Could you check a few things on this model? Use its own coordinates, in mm. Round coordinates to 2 decimals unless told otherwise and drop trailing zeros. Loops run counter-clockwise (first coordinate to the right, second up) from the corner with the lowest first, then second, coordinate; pieces in that order, holes last. Notation, with made-up numbers: (27.5, -7) -> (68.5, -7) arc R29 ccw to (68.5, 18) -> close; hole circle Ø8 at (-23.75, 33.5). An arc over 180 degrees is marked (long way). One line per item, written item: value.
```python
from build123d import *

# Parameters (mm, degrees)
SKETCH2_W           = 90
SKETCH2_H           = 92.5
SKETCH2_R           = 2
SKETCH2_W_2         = 10
SKETCH2_H_2         = 3
SKETCH2_W_3         = 3
SKETCH2_H_3         = 5
SKETCH2_W_4         = 20
SKETCH2_H_4         = 10
BOSS_EXTRUDE1_DEPTH = 3


with BuildPart() as part:
    # Sketch2 → Boss-Extrude1 (new body)
    with BuildSketch(Plane(origin=(0, 0, 0), x_dir=(1, 0, 0), z_dir=(0, 1, 0))):
        Rectangle(SKETCH2_W, SKETCH2_H)
        with Locations((0, -42.25)):
            Circle(SKETCH2_R, mode=Mode.SUBTRACT)
        with Locations((0, 42.25)):
            Circle(SKETCH2_R, mode=Mode.SUBTRACT)
        with Locations((-25, 37.75)):
            Rectangle(SKETCH2_W_2, SKETCH2_H_2, mode=Mode.SUBTRACT)
        with Locations((-40.5, 10.5)):
            Rectangle(SKETCH2_W_3, SKETCH2_H_3, mode=Mode.SUBTRACT)
        with Locations((25, 37.75)):
            Rectangle(SKETCH2_W_2, SKETCH2_H_2, mode=Mode.SUBTRACT)
        with Locations((25, -37.75)):
            Rectangle(SKETCH2_W_2, SKETCH2_H_2, mode=Mode.SUBTRACT)
        with Locations((-25, -37.75)):
            Rectangle(SKETCH2_W_2, SKETCH2_H_2, mode=Mode.SUBTRACT)
        with Locations((-40.5, -10.5)):
            Rectangle(SKETCH2_W_3, SKETCH2_H_3, mode=Mode.SUBTRACT)
        with Locations((40.5, 10.5)):
            Rectangle(SKETCH2_W_3, SKETCH2_H_3, mode=Mode.SUBTRACT)
        with Locations((40.5, -10.5)):
            Rectangle(SKETCH2_W_3, SKETCH2_H_3, mode=Mode.SUBTRACT)
        Rectangle(SKETCH2_W_4, SKETCH2_H_4, mode=Mode.SUBTRACT)
    extrude(amount=BOSS_EXTRUDE1_DEPTH)


solid = part.part
```
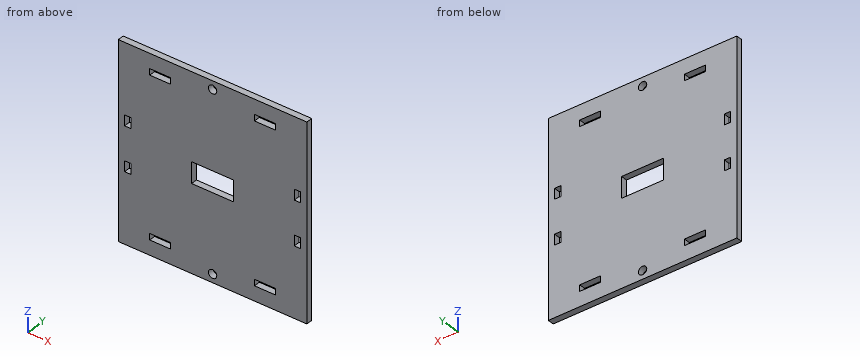
(1) Imagine slicing it at C-C on z = -42.25. Write out the boundary of the cut face in (x, y), then the cut area to 3 significant figures.
Results below:
outline: (-45, 0) -> (-2, 0) -> (-2, 3) -> (-45, 3) -> close; (2, 0) -> (45, 0) -> (45, 3) -> (2, 3) -> close
area: 258 mm²
(2) Imagine slicing it at B-B on x = 0. Write out the boundary of the cut face in (y, z).
Results below:
outline: (0, -46.25) -> (3, -46.25) -> (3, -44.25) -> (0, -44.25) -> close; (0, -40.25) -> (3, -40.25) -> (3, -5) -> (0, -5) -> close; (0, 5) -> (3, 5) -> (3, 40.25) -> (0, 40.25) -> close; (0, 44.25) -> (3, 44.25) -> (3, 46.25) -> (0, 46.25) -> close
(3) For pin 1 Ø3 at (x, z) = (0, -42.25) entering from +Y, with a flat end and sliding along its axis, tell me the tip position at first contact or that it passes through.
Results below:
pin 1: passes through
(4) Imagine slicing it at A-A on x = -26. Write out the boundary of the cut face in (y, z), then the cut area to 4 significant figures.
Results below:
outline: (0, -46.25) -> (3, -46.25) -> (3, -39.25) -> (0, -39.25) -> close; (0, -36.25) -> (3, -36.25) -> (3, 36.25) -> (0, 36.25) -> close; (0, 39.25) -> (3, 39.25) -> (3, 46.25) -> (0, 46.25) -> close
area: 259.5 mm²
(5) Please list where these lines run through material, in increasing order: L1, parallel to Z at x = 0, y = 2.1; L2, parallel to Z at x = 40, y = 1.9; L3, parallel to X at y = 1.55, z = -42.25.
Results below:
L1: z = -46.25 to -44.25, -40.25 to -5, 5 to 40.25, 44.25 to 46.25
L2: z = -46.25 to -13, -8 to 8, 13 to 46.25
L3: x = -45 to -2, 2 to 45
(6) Imagine slicing it at D-D on y = 2.4. Give the number of separate pieces and of enclosed holes in the cut face, then the cut area to 3 significant figures.
Results below:
separate pieces: 1
enclosed holes: 11
area: 7,920 mm²
